The listing builds one solid part. Answer for the finished solid, in the listing's coordinates (mm). Give positions to 0.01 mm unless a question says otherwise; leave off trailing zeros. Write each loop counter-clockwise with the first axis right and the second up, starting at its lowest first coordinate (ties: lowest second). Pieces come first, ordered by that corner, then holes. Notation, with made-up numbers: M 54,-29 L 96,-29 A29 cw 96,4 Z; hole C -3.75,-22.5 d6. An arc over 180 degrees is marked long. Answer as a JSON object with one key per item and string values.
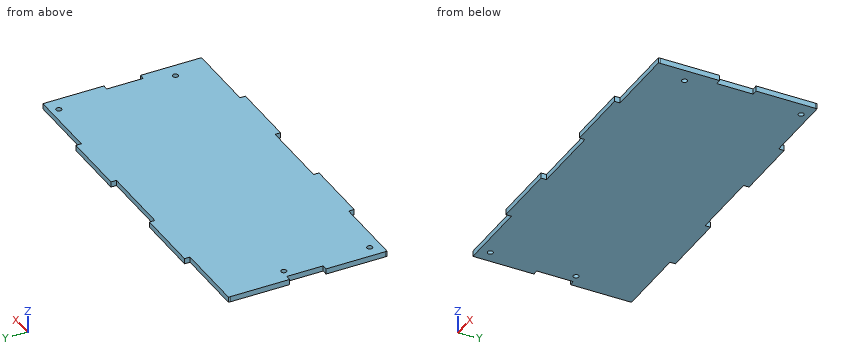
```python
from build123d import *

# Parameters (mm, degrees)
BOSS_EXTRUDE2_DEPTH = 3
SKETCH3_R           = 1.5
SKETCH3_W           = 3
SKETCH3_H           = 20
SKETCH3_W_2         = 40
SKETCH3_H_2         = 3
CUT_EXTRUDE1_DEPTH  = 3


with BuildPart() as part:
    # Sketch1 → Boss-Extrude2 (new body)
    with BuildSketch(Plane.XY):
        with BuildLine():
            Line((-92.5, 46.5), (92.5, 46.5))
            ThreePointArc((92.5, 46.5), (95.328427125, 45.328427125), (96.5, 42.5))
            Line((96.5, 42.5), (96.5, -42.5))
            ThreePointArc((96.5, -42.5), (95.328427125, -45.328427125), (92.5, -46.5))
            Line((92.5, -46.5), (-92.5, -46.5))
            ThreePointArc((-92.5, -46.5), (-95.328427125, -45.328427125), (-96.5, -42.5))
            Line((-96.5, -42.5), (-96.5, 42.5))
            ThreePointArc((-96.5, 42.5), (-95.328427125, 45.328427125), (-92.5, 46.5))
        make_face()
    extrude(amount=BOSS_EXTRUDE2_DEPTH)

    # Sketch3 → Cut-Extrude1 (cut)
    with BuildSketch(Plane.XY.offset(3)):
        with Locations((-88.674, 9.010523044)):
            Circle(SKETCH3_R)
        with Locations((-89.563, -37.598476956)):
            Circle(SKETCH3_R)
        with Locations((88.364, -24.898476956)):
            Circle(SKETCH3_R)
        with Locations((88.491, 38.982523044)):
            Circle(SKETCH3_R)
        with Locations((-95, 0)):
            Rectangle(SKETCH3_W, SKETCH3_H)
        with Locations((95, 0)):
            Rectangle(SKETCH3_W, SKETCH3_H)
        with Locations((76.5, 45)):
            Rectangle(SKETCH3_W_2, SKETCH3_H_2)
        with Locations((-76.5, 45)):
            Rectangle(SKETCH3_W_2, SKETCH3_H_2)
        with Locations((76.5, -45)):
            Rectangle(SKETCH3_W_2, SKETCH3_H_2)
        with Locations((0, 45)):
            Rectangle(SKETCH3_W_2, SKETCH3_H_2)
        with Locations((0, -45)):
            Rectangle(SKETCH3_W_2, SKETCH3_H_2)
        with Locations((-76.5, -45)):
            Rectangle(SKETCH3_W_2, SKETCH3_H_2)
    extrude(amount=-CUT_EXTRUDE1_DEPTH, mode=Mode.SUBTRACT)


solid = part.part
```
1. Consider line 1 along X through (y, z) = (-37.5, 1.95); line 2 along Y through (x, z) = (78.5, 1.9); line 3 along X through (y, z) = (6.5, 0.7). Determine where each line is inside the solid, lowest interval first.
Verdict:
{"line 1": "x = -96.5 to -91.06, -88.07 to 96.5", "line 2": "y = -43.5 to 43.5", "line 3": "x = -93.5 to 93.5"}
2. A cutting plane is placed at B-B, the plane y = -3. Give the vertices of the cut face in (x, z), plus the area to 3 significant figures.
Verdict:
{"outline": "M -93.5,0 L 93.5,0 L 93.5,3 L -93.5,3 Z", "area": "561 mm2"}
3. Flat-ended cylindrical pins translate along their axes: pin 1 (1.5 mm diameter, centred on y = 44.5, z = 2, fed in from +X); pin 2 (0.9 mm diameter, centred on x = 95.5, z = 1.5, fed in from +Y); pin 3 (1.5 mm diameter, centred on y = 45, z = 2, fed in from -X). Find the tip coordinate at first contact, or state that the pin passes through.
Verdict:
{"pin 1": "stops at x = 56.5", "pin 2": "stops at y = 43.5", "pin 3": "stops at x = -56.5"}
4. A cutting plane is placed at A-A, the plane x = -66. Give the vertices of the cut face in (y, z), plus the area to 3 significant figures.
Verdict:
{"outline": "M -43.5,0 L 43.5,0 L 43.5,3 L -43.5,3 Z", "area": "261 mm2"}
5. A cutting plane is placed at C-C, the plane z = 1. Count the separate pieces of the cut face and the enclosed holes in it, plus the area to 3 significant figures.
Verdict:
{"separate pieces": "1", "enclosed holes": "4", "area": "17,100 mm2"}
